```python
from build123d import *

# Parameters (mm, degrees)
SKETCH_1_R      = 1.6
SKETCH_1_R_2    = 1.85
EXTRUDE_1_DEPTH = 3
FILLET_1_R      = 3


with BuildPart() as part:
    # 草图1 → 凸台-拉伸1 (new body)
    with BuildSketch(Plane.XY):
        Polygon((65.759662845, 31.457301477), (53.535196603, 31.457301477), (53.535196603, -19.542698523), (64.984129087, -19.542698523), (113.759662845, -19.542698523), (113.759662845, -29.542698523), (66.535196603, -29.542698523), (66.535196603, -53.542698523), (-13.464803397, -53.542698523), (-13.464803397, 65.457301477), (64.984129087, 65.457301477), (64.984129087, 41.457301477), (114.535196603, 41.457301477), (114.535196603, 31.457301477), align=None)
        with Locations((15.759662845, 60.457301477)):
            Circle(SKETCH_1_R, mode=Mode.SUBTRACT)
        with Locations((35.759662845, 60.457301477)):
            Circle(SKETCH_1_R, mode=Mode.SUBTRACT)
        with Locations((15.759662845, -48.542698523)):
            Circle(SKETCH_1_R, mode=Mode.SUBTRACT)
        with Locations((35.759662845, -48.542698523)):
            Circle(SKETCH_1_R, mode=Mode.SUBTRACT)
        with Locations((-3.464803397, 48.957301477)):
            Circle(SKETCH_1_R, mode=Mode.SUBTRACT)
        with Locations((28.535196603, 48.957301477)):
            Circle(SKETCH_1_R, mode=Mode.SUBTRACT)
        with Locations((-3.464803397, -37.042698523)):
            Circle(SKETCH_1_R, mode=Mode.SUBTRACT)
        with Locations((28.535196603, -37.042698523)):
            Circle(SKETCH_1_R, mode=Mode.SUBTRACT)
        with Locations((62.035196603, -23.042698523)):
            Circle(SKETCH_1_R_2, mode=Mode.SUBTRACT)
        with Locations((106.035196603, -23.042698523)):
            Circle(SKETCH_1_R_2, mode=Mode.SUBTRACT)
        with Locations((62.035196603, 34.957301477)):
            Circle(SKETCH_1_R_2, mode=Mode.SUBTRACT)
        with Locations((106.035196603, 34.957301477)):
            Circle(SKETCH_1_R_2, mode=Mode.SUBTRACT)
        with BuildLine():
            Line((9.302741514, -34.092463325), (15.759662845, -34.092463325))
            ThreePointArc((15.759662845, -34.092463325), (20.759662845, -39.092463325), (15.759662845, -44.092463325))
            Line((15.759662845, -44.092463325), (9.302741514, -44.092463325))
            ThreePointArc((9.302741514, -44.092463325), (4.302741514, -39.092463325), (9.302741514, -34.092463325))
        make_face(mode=Mode.SUBTRACT)
        with BuildLine():
            Line((-1.964803397, 30.957301477), (-1.964803397, 26.957301477))
            ThreePointArc((-1.964803397, 26.957301477), (-3.464803397, 25.457301477), (-4.964803397, 26.957301477))
            Line((-4.964803397, 26.957301477), (-4.964803397, 30.957301477))
            ThreePointArc((-4.964803397, 30.957301477), (-3.464803397, 32.457301477), (-1.964803397, 30.957301477))
        make_face(mode=Mode.SUBTRACT)
        with BuildLine():
            Line((-1.964803397, -15.042698523), (-1.964803397, -19.042698523))
            ThreePointArc((-1.964803397, -19.042698523), (-3.464803397, -20.542698523), (-4.964803397, -19.042698523))
            Line((-4.964803397, -19.042698523), (-4.964803397, -15.042698523))
            ThreePointArc((-4.964803397, -15.042698523), (-3.464803397, -13.542698523), (-1.964803397, -15.042698523))
        make_face(mode=Mode.SUBTRACT)
        with BuildLine():
            Line((27.035196603, -15.042698523), (27.035196603, -19.042698523))
            ThreePointArc((27.035196603, -19.042698523), (28.535196603, -20.542698523), (30.035196603, -19.042698523))
            Line((30.035196603, -19.042698523), (30.035196603, -15.042698523))
            ThreePointArc((30.035196603, -15.042698523), (28.535196603, -13.542698523), (27.035196603, -15.042698523))
        make_face(mode=Mode.SUBTRACT)
        with BuildLine():
            Line((27.035196603, 30.957301477), (27.035196603, 26.957301477))
            ThreePointArc((27.035196603, 26.957301477), (28.535196603, 25.457301477), (30.035196603, 26.957301477))
            Line((30.035196603, 26.957301477), (30.035196603, 30.957301477))
            ThreePointArc((30.035196603, 30.957301477), (28.535196603, 32.457301477), (27.035196603, 30.957301477))
        make_face(mode=Mode.SUBTRACT)
    extrude(amount=EXTRUDE_1_DEPTH)

    # 圆角1
    fillet_1_edges = [part.edges().sort_by_distance(p)[0] for p in [
        (-13.464803397, 65.457301477, 1.5),
        (64.984129087, 65.457301477, 1.5),
        (64.984129087, 41.457301477, 1.5),
        (114.535196603, 41.457301477, 1.5),
        (113.759662845, -29.542698523, 1.5),
        (66.535196603, -29.542698523, 1.5),
        (66.535196603, -53.542698523, 1.5),
        (-13.464803397, -53.542698523, 1.5),
    ]]
    fillet(fillet_1_edges, radius=FILLET_1_R)


solid = part.part
```
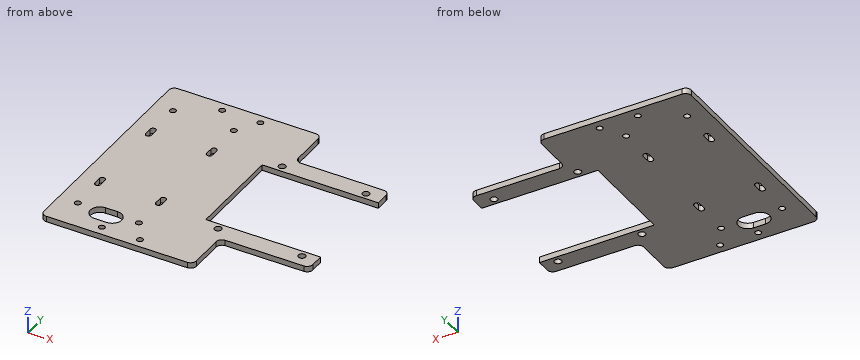
Model file for the job. Use its own axes, mm. Round coordinates to 2 decimals unless told otherwise and drop trailing zeros. Write each loop counter-clockwise with the first axis right and the second up, starting at its lowest first coordinate (ties: lowest second). Pieces come first, ordered by that corner, then holes. Notation, with made-up numbers: (56, 69.5) - (73, 69.5) arc R27 cw to (73, 102.5) - close; hole circle Ø8 at (78, -35.75). An arc over 180 degrees is marked (long way). One line per item, written item: value.
(1) Cut at A-A, the plane x = 89.5. Give the cut face in (y, z), plus the area to 3 significant figures.
Values follow:
outline: (-29.54, 0) - (-19.54, 0) - (-19.54, 3) - (-29.54, 3) - close; (31.46, 0) - (41.46, 0) - (41.46, 3) - (31.46, 3) - close
area: 60.0 mm²
(2) Drop flat-ended pins along their axis: P1, Ø0.9, axis at y = 29.5, z = 1.5, coming from the +X side; P2, Ø1.5, axis at x = 85.5, z = 0.5, coming from the -Y side. Give the stop position or say it passes through.
Values follow:
P1: stops at x = 53.54
P2: stops at y = -29.54
(3) Cut at B-B, the plane z = 2.25. Give the number of separate pieces and of enclosed holes in the cut face, plus the area to 3 significant figures.
Values follow:
separate pieces: 1
enclosed holes: 17
area: 9,440 mm²
(4) Cut at D-D, the plane y = 53. Give the cut face in (x, z), plus the area to 3 significant figures.
Values follow:
outline: (-13.46, 0) - (64.98, 0) - (64.98, 3) - (-13.46, 3) - close
area: 235 mm²
(5) Cut at C-C, the plane y = 17. Give the cut face in (x, z), plus the area to 3 significant figures.
Values follow:
outline: (-13.46, 0) - (53.54, 0) - (53.54, 3) - (-13.46, 3) - close
area: 201 mm²
(6) Wall check: probe 1 along X at (y, z) = (-19, 2.85); probe 2 along Y at (x, z) = (91, 2.1); probe 3 along X at (y, z) = (35.5, 2.35). Give the ranges that are in metal, low to high.
Values follow:
probe 1: x = -13.46 to -4.96, -1.96 to 27.04, 30.04 to 53.54
probe 2: y = -29.54 to -19.54, 31.46 to 41.46
probe 3: x = -13.46 to 60.27, 63.8 to 104.27, 107.8 to 114.54
